from build123d import *

# Parameters (mm, degrees)
F0_W      = 58.02
F0_H      = 96.3
F1_DEPTH  = 5.5
F2_W      = 43.42
F2_H      = 81.7
F3_DEPTH  = 5.501
F4_W      = 2.4
F4_H      = 85.75
F5_DEPTH  = 54.5
F6_DEPTH  = 9
F7_R      = 2.5
F8_DEPTH  = 5.501
F9_DEPTH  = 16
F10_W     = 47
F10_H     = 3.25
F11_DEPTH = 19
F13_DEPTH = 0.4
F14_DEPTH = 3.25
F15_DEPTH = 2
F16_DEPTH = 2
F12_R     = 2.4
F17_DEPTH = 2
F18_R     = 0.5
F19_DEPTH = 0.3
F20_DEPTH = 1.5
F21_DEPTH = 1.5
F22_DEPTH = 0.2


with BuildPart() as f1:
    # F0 (on Front) → F1 (new body)
    with BuildSketch(Plane.XZ):
        Rectangle(F0_W, F0_H)
    extrude(amount=F1_DEPTH)

    # F2 (on face) → F3 (cut, through all)
    with BuildSketch(Plane.XZ.offset(5.5)):
        Rectangle(F2_W, F2_H)
    extrude(amount=-F3_DEPTH, mode=Mode.SUBTRACT)

    # F4 (on face) → F5 (cut)
    with BuildSketch(Plane.YZ.offset(29.01)):
        with Locations((-2.6675368889, 0)):
            Rectangle(F4_W, F4_H)
    extrude(amount=-F5_DEPTH, mode=Mode.SUBTRACT)

    # F6 (add): a face of the model
    f6_faces = [f1.faces().sort_by_distance(p)[0] for p in [
        (0, -2.75, 48.15),
    ]]
    extrude(f6_faces, amount=F6_DEPTH)

    # F7 (on face) → F8 (cut, through all)
    with BuildSketch(Plane.XZ.offset(5.5)):
        with Locations((0, 49.4283474982)):
            Circle(F7_R)
    extrude(amount=-F8_DEPTH, mode=Mode.SUBTRACT)

    # F9 (add): a face of the model
    f9_faces = [f1.faces().sort_by_distance(p)[0] for p in [
        (0, -2.75, -48.15),
    ]]
    extrude(f9_faces, amount=F9_DEPTH)

    # F10 (on face) → F11 (cut)
    with BuildSketch(Plane(origin=(0, 0, -64.15), x_dir=(1, 0, 0), z_dir=(0, 0, -1))):
        with Locations((0, 2.75)):
            Rectangle(F10_W, F10_H)
    extrude(amount=-F11_DEPTH, mode=Mode.SUBTRACT)

    # F13 (cut): a face of the model
    f13_faces = [f1.faces().sort_by_distance(p)[0] for p in [
        (1.76, -2.6675368889, 42.875),
    ]]
    extrude(f13_faces, amount=-F13_DEPTH, mode=Mode.SUBTRACT)

    # F14 (cut): a face of the model
    f14_faces = [f1.faces().sort_by_distance(p)[0] for p in [
        (-28.4271989705, -2.75, -64.15),
    ]]
    extrude(f14_faces, amount=-F14_DEPTH, mode=Mode.SUBTRACT)

    # F15 (cut): a face of the model
    f15_faces = [f1.faces().sort_by_distance(p)[0] for p in [
        (23.5, -2.75, -53.025),
    ]]
    extrude(f15_faces, amount=-F15_DEPTH, mode=Mode.SUBTRACT)

    # F16 (cut): a face of the model
    f16_faces = [f1.faces().sort_by_distance(p)[0] for p in [
        (-23.5, -2.75, -53.025),
    ]]
    extrude(f16_faces, amount=-F16_DEPTH, mode=Mode.SUBTRACT)

    # F12 (on face) → F17 (join)
    with BuildSketch(Plane.XZ.offset(1.125)):
        with Locations((-16.5364966542, -54.65)):
            Circle(F12_R)
    extrude(amount=F17_DEPTH)

    # F18
    f18_edges = [f1.edges().sort_by_distance(p)[0] for p in [
        (-18.936497, -3.125, -54.65),
    ]]
    fillet(f18_edges, radius=F18_R)

    # F19 (cut): a face of the model
    f19_faces = [f1.faces().sort_by_distance(p)[0] for p in [
        (27.990584849, -3.8675368889, 0.2),
    ]]
    extrude(f19_faces, amount=-F19_DEPTH, mode=Mode.SUBTRACT)

    # F20 (add): a face of the model
    f20_faces = [f1.faces().sort_by_distance(p)[0] for p in [
        (27.6946246581, 0, -1.875),
    ]]
    extrude(f20_faces, amount=F20_DEPTH)

    # F21 (add): a face of the model
    f21_faces = [f1.faces().sort_by_distance(p)[0] for p in [
        (27.6946246581, -5.5, -1.875),
    ]]
    extrude(f21_faces, amount=F21_DEPTH)

    # F22 (cut): a face of the model
    f22_faces = [f1.faces().sort_by_distance(p)[0] for p in [
        (0, -4.375, -53.025),
    ]]
    extrude(f22_faces, amount=-F22_DEPTH, mode=Mode.SUBTRACT)


solid = f1.part
Design review of the part built by this model. Coordinates are the model's own, in mm. A direction names the side the tool comes from. Coordinates: 2 decimals unless noted, no trailing zeros. Write each loop counter-clockwise with the first axis right and the second up, starting at its lowest first coordinate (ties: lowest second). Pieces come first, ordered by that corner, then holes. Notation, with made-up numbers: (-17.75, 64) - (0.25, 64) arc R20 ccw to (0.25, 97) - close; hole circle Ø4 at (26.5, -5.5). An arc over 180 degrees is marked (long way). Use one line per item in the form item = value.
Q1. Consider section D-D (z = 25.5). Write out the cut boundary in (x, y).
Taken from the geometry:
outline = (-29.01, -7) - (-21.71, -7) - (-21.71, -4.17) - (-25.49, -4.17) - (-25.49, -1.47) - (-21.71, -1.47) - (-21.71, 1.5) - (-29.01, 1.5) - close; (21.71, -7) - (29.01, -7) - (29.01, -4.17) - (21.71, -4.17) - close; (21.71, -1.47) - (29.01, -1.47) - (29.01, 1.5) - (21.71, 1.5) - close
Q2. Consider section A-A (z = -54.65). Write out the cut boundary in (x, y) (1 decimal).
Taken from the geometry:
outline = (-29, -7) - (29, -7) - (29, 1.5) - (-29, 1.5) - close; hole (-25.5, -4.6) - (25.5, -4.6) - (25.5, -1.1) - (-14.1, -1.1) - (-14.1, -2.6) arc R0.5 cw to (-14.6, -3.1) - (-18.4, -3.1) arc R0.5 cw to (-18.9, -2.6) - (-18.9, -1.1) - (-25.5, -1.1) - close
Q3. The part is to be moulded in two halves that separate along Z. For faces 4 (the flat face through (-29.01, -3, -3)), 5 (the flat face through (21.71, 0, -1)), 6 (the flat face through (0, -5, -60.9)), say which applies: +Z half, -Z half, draft (parallel to the pull), parting line (faces both ways), or undercut.
Taken from the geometry:
face_4 = draft
face_5 = undercut
face_6 = -Z half
Q4. Machinability: for faces 1 (the flat face through (0, -4.575, -53)), 2 (the cylindrical face through (-17.057, -1.864, -56.993)), 3 (the flat face through (21.71, -6, -1)), which of the approach directions +Z, -Z, +X, -X, +Y, -Y give a long, thin tool a straight path to every point of the face, cutting with its end or side? Answer none if there is none.
Taken from the geometry:
face_1 = -Z
face_2 = none
face_3 = +Y, -Y
Q5. Consider section C-C (x = -20.5). Write out the cut boundary in (y, z) (3 decimals), plus the area to 3 significant figures.
Taken from the geometry:
outline = (-7, -60.9) - (-4.575, -60.9) - (-4.575, -45.15) - (-1.125, -45.15) - (-1.125, -60.9) - (1.5, -60.9) - (1.5, -40.85) - (-1.468, -40.85) - (-1.468, -42.875) - (-4.168, -42.875) - (-4.168, -40.85) - (-7, -40.85) - close; (-7, 40.85) - (-4.168, 40.85) - (-4.168, 43.275) - (-1.468, 43.275) - (-1.468, 40.85) - (1.5, 40.85) - (1.5, 57.15) - (-7, 57.15) - close
area = 243 mm^2
Q6. Insertion check: pin 1 Ø3 at (x, z) = (0, 49.43) entering from -Y; pin 2 Ø0.8 at (x, y) = (-1.5, -3) entering from -Z; pin 3 Ø0.8 at (y, z) = (-2.5, 8.5) entering from +X. Each pin has a flat end and moves straight along its axis. Give the tip position at first contact, or say it passes through.
Taken from the geometry:
pin_1 = through
pin_2 = -45.15
pin_3 = -25.49
Q7. Consider section B-B (x = 23). Write out the cut boundary in (y, z) (3 decimals), plus the area to 3 significant figures.
Taken from the geometry:
outline = (-7, -60.9) - (-4.575, -60.9) - (-4.575, -45.15) - (-1.125, -45.15) - (-1.125, -60.9) - (1.5, -60.9) - (1.5, 57.15) - (-7, 57.15) - close; hole (-4.168, -42.875) - (-1.468, -42.875) - (-1.468, 43.275) - (-4.168, 43.275) - close
area = 716 mm^2
Q8. For probe 1 along Z at (x, y) = (0, -3.25) (3 decimals); probe 2 along Z at (x, y) = (0, -6.3); probe 3 along Z at (x, y) = (-14, -2.25) (3 decimals), list the stretches that pass through material, from the lowest coordinate up.
Taken from the geometry:
probe_1 = -45.15 to -42.875, 43.275 to 46.928, 51.928 to 57.15
probe_2 = -60.9 to -40.85, 40.85 to 46.93, 51.93 to 57.15
probe_3 = -45.15 to -42.875, 43.275 to 57.15
